from build123d import *

# Parameters (mm, degrees)
ESQUISSE1_W             = 455
ESQUISSE1_H             = 250
ESQUISSE1_R             = 6.5
BOSS_EXTRU_1_DEPTH      = 3
ESQUISSE4_W             = 100
ESQUISSE4_H             = 25
ESQUISSE4_W_2           = 38
ESQUISSE4_H_2           = 84
ESQUISSE4_W_3           = 10
ESQUISSE4_H_3           = 44
ENL_V_MAT_EXTRU_3_DEPTH = 10
CONG_1_R                = 2


with BuildPart() as part:
    # Esquisse1 → Boss.-Extru.1 (new body)
    with BuildSketch(Plane.XY):
        Rectangle(ESQUISSE1_W, ESQUISSE1_H)
        with Locations((106.5, 95)):
            Circle(ESQUISSE1_R, mode=Mode.SUBTRACT)
        with Locations((202.5, 95)):
            Circle(ESQUISSE1_R, mode=Mode.SUBTRACT)
        with Locations((106.5, -105)):
            Circle(ESQUISSE1_R, mode=Mode.SUBTRACT)
        with Locations((202.5, -105)):
            Circle(ESQUISSE1_R, mode=Mode.SUBTRACT)
        with Locations((-103.5, -105)):
            Circle(ESQUISSE1_R, mode=Mode.SUBTRACT)
        with Locations((-103.5, 95)):
            Circle(ESQUISSE1_R, mode=Mode.SUBTRACT)
        with Locations((-199.5, 95)):
            Circle(ESQUISSE1_R, mode=Mode.SUBTRACT)
        with Locations((-199.5, -105)):
            Circle(ESQUISSE1_R, mode=Mode.SUBTRACT)
    extrude(amount=BOSS_EXTRU_1_DEPTH)

    # Esquisse4 → Enlèv. mat.-Extru.3 (cut)
    with BuildSketch(Plane.XY.offset(3)):
        with Locations((-177.5, -30.5)):
            Rectangle(ESQUISSE4_W, ESQUISSE4_H)
        with Locations((-37.5, -83)):
            Rectangle(ESQUISSE4_W_2, ESQUISSE4_H_2)
        with Locations((222.5, -63)):
            Rectangle(ESQUISSE4_W_3, ESQUISSE4_H_3)
    extrude(amount=-ENL_V_MAT_EXTRU_3_DEPTH, mode=Mode.SUBTRACT)

    # Congé1
    cong_1_edges = [part.edges().sort_by_distance(p)[0] for p in [
        (-127.5, -18, 1.5),
        (-127.5, -43, 1.5),
        (-56.5, -41, 1.5),
        (-18.5, -41, 1.5),
    ]]
    fillet(cong_1_edges, radius=CONG_1_R)


solid = part.part
Here's how the part is built. I have some questions about the finished solid (model axes, mm). Round coordinates to 2 decimals unless told otherwise and drop trailing zeros. Order: outer loops, then holes, each group sorted by start corner. A loop starts at its lowest first (then second) coordinate and runs counter-clockwise, first axis right, second up. Notation, with made-up numbers: M -38.5,15 L -22.5,15 A6 cw -22.5,21 Z; hole C 19,52 d7. An arc over 180 degrees is marked long. Return JSON: item names as keys, results as strings. Group by question number.
1. I'm going to push flat-ended pins straight in: pin 1 Ø1.5 at (x, z) = (-41.5, 2) entering from -Y; pin 2 Ø0.9 at (y, z) = (-26.5, 1) entering from -X. Where does each tip first touch, or does it pass through?
2. If we section it at C-C on y = -105: List the corners of the cut face in (x, z) for me.
3. If we section it at A-A on x = 106.5: List the corners of the cut face in (y, z) for me, then the cut area to 3 significant figures.
4. Please list where these lines run through material, in increasing order: probe 1 along Y at (x, z) = (-199.5, 2.35); probe 2 along Y at (x, z) = (106.5, 1.4); probe 3 along Y at (x, z) = (-134.5, 0.4).
5. If we mould it in two halves opening along Y, with no side actions, what happens to faces 1 (the face through (-204.658, -108.955, 1.479)), 2 (the face through (-3, 2, 3))? For each: pulls with the +Y half, pulls with the -Y half, needs draft (parallel to the pull), parting line crosses it, or undercut.
6. If we section it at B-B on y = 95: List the corners of the cut face in (x, z) for me, then the cut area to 3 significant figures.
7. If we section it at D-D on x = -186: List the corners of the cut face in (y, z) for me.
Reply:
{
 "1": {"pin 1": "y = -41", "pin 2": "x = -127.5"},
 "2": {"outline": "M -227.5,0 L -206,0 L -206,3 L -227.5,3 Z; M -193,0 L -110,0 L -110,3 L -193,3 Z; M -97,0 L -56.5,0 L -56.5,3 L -97,3 Z; M -18.5,0 L 100,0 L 100,3 L -18.5,3 Z; M 113,0 L 196,0 L 196,3 L 113,3 Z; M 209,0 L 227.5,0 L 227.5,3 L 209,3 Z"},
 "3": {"outline": "M -125,0 L -111.5,0 L -111.5,3 L -125,3 Z; M -98.5,0 L 88.5,0 L 88.5,3 L -98.5,3 Z; M 101.5,0 L 125,0 L 125,3 L 101.5,3 Z", "area": "672 mm^2"},
 "4": {"probe 1": "-125 to -111.5, -98.5 to -43, -18 to 88.5, 101.5 to 125", "probe 2": "-125 to -111.5, -98.5 to 88.5, 101.5 to 125", "probe 3": "-125 to -43, -18 to 125"},
 "5": {"face 1": "undercut", "face 2": "needs draft"},
 "6": {"outline": "M -227.5,0 L -206,0 L -206,3 L -227.5,3 Z; M -193,0 L -110,0 L -110,3 L -193,3 Z; M -97,0 L 100,0 L 100,3 L -97,3 Z; M 113,0 L 196,0 L 196,3 L 113,3 Z; M 209,0 L 227.5,0 L 227.5,3 L 209,3 Z", "area": "1,210 mm^2"},
 "7": {"outline": "M -125,0 L -43,0 L -43,3 L -125,3 Z; M -18,0 L 125,0 L 125,3 L -18,3 Z"}
}
